Build history of the part. All positions in model axes, mm. Face numbers are marked on the shaded views. A direction names the side the tool comes from. Round coordinates to 2 decimals unless told otherwise and drop trailing zeros. Write each loop counter-clockwise with the first axis right and the second up, starting at its lowest first coordinate (ties: lowest second). Pieces come first, ordered by that corner, then holes. Notation, with made-up numbers: (-8, 42.25) -> (11, 42.25) arc R27 ccw to (11, 81.25) -> close; hole circle Ø10 at (-38.75, -10.5). An arc over 180 degrees is marked (long way). Answer as CSV lines item,"result".
from build123d import *

# Parameters (mm, degrees)
BOSS_EXTRUDE1_DEPTH = 10
SKETCH3_R           = 2.45
CUT_EXTRUDE1_DEPTH  = 11
SKETCH4_R           = 1.6
CUT_EXTRUDE2_DEPTH  = 5
CUT_EXTRUDE3_START  = -5
SKETCH5_R           = 1.6
CUT_EXTRUDE3_DEPTH  = 5
SKETCH6_W           = 12.5
SKETCH6_H           = 1.6
CUT_EXTRUDE4_DEPTH  = 11
FILLET1_R           = 1


with BuildPart() as part:
    # Sketch2 → Boss-Extrude1 (new body)
    with BuildSketch(Plane.XY):
        with BuildLine():
            Line((7.861835452, 3.19), (-7.738161553, 3.19))
            Line((-7.738161553, 3.19), (-31.1, 3.19))
            Line((-31.1, 3.19), (-31.1, 2.34))
            ThreePointArc((-31.1, 2.34), (-31.290380592, 1.880380592), (-31.75, 1.69))
            Line((-31.75, 1.69), (-32.1, 1.69))
            Line((-32.1, 1.69), (-32.1, -3.51))
            Line((-32.1, -3.51), (-28.800002213, -3.51))
            Line((-28.800002213, -3.51), (-28.800002213, -4.51))
            Line((-28.800002213, -4.51), (-22.200001624, -4.51))
            Line((-22.200001624, -4.51), (-22.200001624, -3.51))
            Line((-22.200001624, -3.51), (-16.749999161, -3.51))
            Line((-16.749999161, -3.51), (-16.749999161, -4.51))
            Line((-16.749999161, -4.51), (-10.149998572, -4.51))
            Line((-10.149998572, -4.51), (-10.149998572, -3.51))
            Line((-10.149998572, -3.51), (10.25999916, -3.51))
            Line((10.25999916, -3.51), (10.25999916, -4.51))
            Line((10.25999916, -4.51), (16.85999975, -4.51))
            Line((16.85999975, -4.51), (16.85999975, -3.51))
            Line((16.85999975, -3.51), (22.200001602, -3.51))
            Line((22.200001602, -3.51), (22.200001602, -4.51))
            Line((22.200001602, -4.51), (28.800002191, -4.51))
            Line((28.800002191, -4.51), (28.800002191, -3.51))
            Line((28.800002191, -3.51), (32.1, -3.51))
            Line((32.1, -3.51), (32.1, 1.69))
            Line((32.1, 1.69), (31.75, 1.69))
            ThreePointArc((31.75, 1.69), (31.290380592, 1.880380592), (31.1, 2.34))
            Line((31.1, 2.34), (31.1, 3.19))
            Line((31.1, 3.19), (7.861835452, 3.19))
        make_face()
    extrude(amount=BOSS_EXTRUDE1_DEPTH)

    # Sketch3 → Cut-Extrude1 (cut)
    with BuildSketch(Plane.XY.offset(10)):
        with Locations((-20, 0)):
            Circle(SKETCH3_R)
        with Locations((-12, 0)):
            Circle(SKETCH3_R)
        with Locations((12, 0)):
            Circle(SKETCH3_R)
        with Locations((20, 0)):
            Circle(SKETCH3_R)
    extrude(amount=-CUT_EXTRUDE1_DEPTH, mode=Mode.SUBTRACT)

    # Sketch4 → Cut-Extrude2 (cut)
    with BuildSketch(Plane(origin=(32.1, 0, 0), x_dir=(0, 0, -1), z_dir=(1, 0, 0))):
        with Locations((-5, -0.91)):
            Circle(SKETCH4_R)
    extrude(amount=-CUT_EXTRUDE2_DEPTH, mode=Mode.SUBTRACT)

    # Sketch5 → Cut-Extrude3 (cut)
    with BuildSketch(Plane.ZY.offset(32.1).offset(CUT_EXTRUDE3_START)):
        with Locations(Location((5, -0.91, 0), (0, 0, 180))):
            Circle(SKETCH5_R)
    extrude(amount=CUT_EXTRUDE3_DEPTH, mode=Mode.SUBTRACT)

    # Sketch6 → Cut-Extrude4 (cut)
    with BuildSketch(Plane.XY.offset(10)):
        with Locations((0, 2.39)):
            Rectangle(SKETCH6_W, SKETCH6_H)
    extrude(amount=-CUT_EXTRUDE4_DEPTH, mode=Mode.SUBTRACT)

    # Fillet1
    fillet1_edges = [part.edges().sort_by_distance(p)[0] for p in [
        (6.25, 3.19, 5),
        (-6.25, 3.19, 5),
    ]]
    fillet(fillet1_edges, radius=FILLET1_R)


solid = part.part
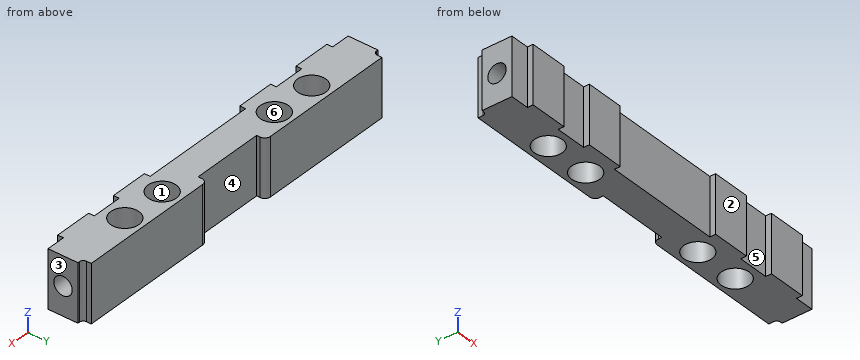
1. Cut at A-A, the plane x = 12. Write the cut outline in (y, z).
Results found:
outline,"(-4.51, 0) -> (-2.45, 0) -> (-2.45, 10) -> (-4.51, 10) -> close; (2.45, 0) -> (3.19, 0) -> (3.19, 10) -> (2.45, 10) -> close"
2. Cut at D-D, the plane z = 5. Count the separate pieces of the cut face and the enclosed holes in it, then the cut area to 3 significant figures.
Results found:
separate pieces,"1"
enclosed holes,"4"
area,"326 mm2"
3. Which spindle directions (+Z, -Z, +X, -X, +Y, -Y) get a long thin tool onto all of the face, cutting with end or side? Do the marked faces 4, 5 and 6. Say none if no direction does.
Results found:
face 4,"+Z, -Z, +Y"
face 5,"+Z, -Z, -Y"
face 6,"+Z, -Z"
4. Cut at C-C, the plane x = 20. Write the cut outline in (y, z), then the cut area to 3 significant figures.
Results found:
outline,"(-3.51, 0) -> (-2.45, 0) -> (-2.45, 10) -> (-3.51, 10) -> close; (2.45, 0) -> (3.19, 0) -> (3.19, 10) -> (2.45, 10) -> close"
area,"18.0 mm2"
5. Probe line 1 along X through (y, z) = (-4, 9.5); line 2 along Y through (x, z) = (28.35, 5); line 3 along Y through (x, z) = (-12, 3). List the from-to ranges inside material, lowest first.
Results found:
line 1,"x = -28.8 to -22.2, -16.75 to -10.15, 10.26 to 16.86, 22.2 to 28.8"
line 2,"y = -4.51 to -2.51, 0.69 to 3.19"
line 3,"y = -4.51 to -2.45, 2.45 to 3.19"
6. Drop flat-ended pins along their axis: pin 1 Ø2 at (y, z) = (-1, 4.5) entering from -X; pin 2 Ø0.5 at (y, z) = (-4, 3) entering from -X; pin 3 Ø1 at (x, z) = (-1, 8.5) entering from -Y. Give the stop position or say it passes through.
Results found:
pin 1,"stops at x = -27.1"
pin 2,"stops at x = -28.8"
pin 3,"stops at y = -3.51"
7. Cut at B-B, the plane y = -0.91. Write the cut outline in (x, z).
Results found:
outline,"(-32.1, 0) -> (-22.27, 0) -> (-22.27, 10) -> (-32.1, 10) -> (-32.1, 6.6) -> (-27.1, 6.6) -> (-27.1, 3.4) -> (-32.1, 3.4) -> close; (-17.73, 0) -> (-14.27, 0) -> (-14.27, 10) -> (-17.73, 10) -> close; (-9.73, 0) -> (9.73, 0) -> (9.73, 10) -> (-9.73, 10) -> close; (14.27, 0) -> (17.73, 0) -> (17.73, 10) -> (14.27, 10) -> close; (22.27, 0) -> (32.1, 0) -> (32.1, 3.4) -> (27.1, 3.4) -> (27.1, 6.6) -> (32.1, 6.6) -> (32.1, 10) -> (22.27, 10) -> close"
8. Mould opens along X. For the marked faces 1, 2 and 3 say: +X half, -X half, draft (parallel to the pull), parting line (faces both ways), or undercut.
Results found:
face 1,"undercut"
face 2,"draft"
face 3,"+X half"
